The model under review builds one solid part; all positions refer to its coordinate system, in mm. A direction names the side the tool comes from. Round coordinates to 2 decimals unless told otherwise and drop trailing zeros. Loops run counter-clockwise (first coordinate to the right, second up) from the corner with the lowest first, then second, coordinate; pieces in that order, holes last. Notation, with made-up numbers: M 78,14 L 122,14 A23 ccw 122,28 Z; hole C -3,56 d3. An arc over 180 degrees is marked long. Return JSON: item names as keys, results as strings. Group by question number.
Q1. Clearance check with a flat-ended pin moving along its axis: pin 1 Ø2 at (x, z) = (356.5, -52) entering from -Y. State where the tip first meets the part, or that it passes through.
Q2. Consider section C-C (y = 39.5). State the section outline as (x, z) points.
Q3. To check wall thickness, follow line 1 along X through (y, z) = (205, -39); line 2 along Y through (x, z) = (231, -59.5); line 3 along Y through (x, z) = (612, 65). State the ranges of each line that lie inside material, in increasing order.
Q4. For faces 1 (the face through (456, 390, 6)), 2 (the face through (456, 400, -1)), 3 (the face through (443.84, 370.74, 57.38)), list the 3-axis set-ups (+Z, -Z, +X, -X, +Y, -Y) from which the entire face can be reached by the end or side of a thin tool; tool diameter is ignored.
Q5. Consider section A-A (z = 55). State the section outline as (x, y) points.
Q6. Consider section B-B (x = 664). State the section outline as (y, z) points.
Q7. Draft analysis for pull direction X (two halves, no side actions). For faces 4 (the face through (900, 197, -1)), 5 (the face through (444, 0, -1)), 6 (the face through (10, 203, 6)), state which applies: pulls with the +X half, pulls with the -X half, needs draft (parallel to the pull), parting line crosses it, or undercut.
Q8. Consider section D-D (z = -24). State the section outline as (x, y) points, and give its area (3 significant figures).
Autodesk Inventor part; units mm, degrees
ref_plane "YZ Plane" through (0, 0, 0) normal (1, 0, 0) x (0, 1, 0)
ref_plane "XZ Plane" through (0, 0, 0) normal (0, 1, 0) x (-1, 0, 0)
ref_plane "XY Plane" through (0, 0, 0) normal (0, 0, 1) x (1, 0, 0)
sketch "스케치1" plane through (0, 0, 0) normal (0, 0, 1) x (1, 0, 0)
  line L0 (0, 0) -> (900, 0)
  line L1 (900, 0) -> (900, 400)
  line L2 (900, 400) -> (0, 400)
  line L3 (0, 400) -> (0, 0)
  dimension "d2" = 900
  dimension "d3" = 400
extrude "돌출1" add sketch "스케치1" along normal mid plane 150
sketch "스케치2" plane through (0, 0, 75) normal (0, 0, 1) x (1, 0, 0)
  line L0 (10, 10) -> (890, 10)
  line L1 (890, 10) -> (890, 390)
  line L2 (890, 390) -> (10, 390)
  line L3 (10, 390) -> (10, 10)
  line L4 (0, 400) -> (0, 0)
  line L5 (900, 400) -> (0, 400)
  line L6 (900, 0) -> (900, 400)
  line L7 (900, 0) -> (0, 0)
  point P0 (0, 200)
  point P1 (10, 200)
  dimension "d6" = 10
  dimension "d7" = 10
  dimension "d8" = 10
  dimension "d10" = 10
extrude "돌출2" cut sketch "스케치2" against normal blind 140 contours L3 L2 L1 L0
sketch "스케치3" plane through (10, 10, 75) normal (1, 0, 0) x (0, 0, -1)
  circle A0 centre (20, 350) radius 11
  line L0 (150, 390) -> (0, 390)
  line L1 (0, 390) -> (0, -10)
  point P0 (75, -10)
  dimension "d13" = 40
  dimension "d14" = 20
  dimension "d15" = 22
extrude "돌출3" add sketch "스케치3" along normal blind 880
properties part number "상자구상도"
Values:
{
 "1": {"pin 1": "stops at y = 0"},
 "2": {"outline": "M 0,-75 L 900,-75 L 900,75 L 890,75 L 890,-65 L 10,-65 L 10,75 L 0,75 Z"},
 "3": {"line 1": "x = 0 to 10, 890 to 900", "line 2": "y = 0 to 10, 390 to 400", "line 3": "y = 0 to 10, 355.42 to 364.58, 390 to 400"},
 "4": {"face 1": "+Z", "face 2": "+Z, -Z, +X, -X, +Y", "face 3": "none"},
 "5": {"outline": "M 0,0 L 900,0 L 900,400 L 0,400 Z; hole M 10,10 L 890,10 L 890,349 L 10,349 Z; hole M 10,371 L 890,371 L 890,390 L 10,390 Z"},
 "6": {"outline": "M 0,-75 L 400,-75 L 400,75 L 390,75 L 390,-65 L 10,-65 L 10,75 L 0,75 Z; C 360,55 d22"},
 "7": {"face 4": "pulls with the +X half", "face 5": "needs draft", "face 6": "undercut"},
 "8": {"outline": "M 0,0 L 900,0 L 900,400 L 0,400 Z; hole M 10,10 L 890,10 L 890,390 L 10,390 Z", "area": "25,600 mm2"}
}
